Autodesk Fusion 360 part; units mm, degrees
sketch "Sketch1" plane through (0, 0, 0) normal (0, 0, 1) x (1, 0, 0)
  line L0 (0, 0) -> (-200, 0)
  line L1 (-200, 0) -> (-200, 25)
  line L2 (-200, 25) -> (0, 25)
  line L3 (0, 25) -> (0, 0)
extrude "Extrude1" add sketch "Sketch1" along normal blind 30
ref_plane "WorkPlane2" through (-100, 12.5, 15) normal (1, 0, 0) x (0, 1, 0)
sketch "Sketch2" plane through (0, 0, 0) normal (0, -1, 0) x (1, 0, 0)
  line L0 (-200, 0) -> (0, 0)
  line L1 (0, 0) -> (0, 30)
  line L2 (0, 30) -> (-200, 30)
  line L3 (-200, 30) -> (-200, 0)
ref_plane "WorkPlane1" through (-100, 12.5, 15) normal (0, 0, 1) x (1, 0, 0)
sketch "Sketch3" plane through (0, 0, 15) normal (0, 0, 1) x (1, 0, 0)
  line L0 (-200, 25) -> (-180, 25)
  line L1 (-180, 25) -> (-180, 0)
  line L2 (-180, 0) -> (-200, 0)
  line L3 (-200, 0) -> (-200, 25)
extrude "Extrude2" cut 1 faces at (-200, 8.3333, 20) along direction (1, 0, 0) blind 1
sketch "Sketch4" plane through (0, 0, 30) normal (0, 0, 1) x (-1, 0, 0)
  line L0 (0, -25) -> (199, -25)
  line L1 (199, 0) -> (0, 0)
  line L2 (0, 0) -> (22, 0)
  line L3 (22, 0) -> (22, -25)
  line L4 (22, -25) -> (0, -25)
  line L5 (0, -25) -> (0, 0)
  line L6 (199, -25) -> (199, 0)
  line L7 (0, 0) -> (0, -25)
extrude "Extrude3" cut sketch "Sketch4" against normal blind 6 contours L0 L1 L2 L3 L4 L5 L7
sketch "Sketch5" plane through (0, 0, 0) normal (0, 0, -1) x (1, 0, 0)
  line L0 (0, 0) -> (-199, 0)
  line L1 (-199, -25) -> (0, -25)
  line L2 (0, 0) -> (-22, 0)
  line L3 (-22, 0) -> (-22, -25)
  line L4 (-22, -25) -> (0, -25)
  line L5 (0, -25) -> (0, 0)
  line L6 (-199, 0) -> (-199, -25)
  line L7 (0, -25) -> (0, 0)
extrude "Extrude4" cut sketch "Sketch5" against normal blind 6 contours L0 L1 L2 L3 L4 L5 L7
sketch "Sketch6" plane through (0, 0, 30) normal (0, 0, 1) x (-1, 0, 0)
  line L0 (199, 0) -> (22, 0)
  line L1 (22, 0) -> (22, -25)
  line L2 (22, -25) -> (199, -25)
  line L3 (34.9313, -5) -> (165.0687, -5)
  line L4 (165.0687, -5) -> (165.0687, -20)
  line L5 (165.0687, -20) -> (34.9313, -20)
  line L6 (34.9313, -20) -> (34.9313, -5)
  line L7 (199, -25) -> (199, 0)
extrude "Extrude5" cut sketch "Sketch6" against normal blind 43 contours L3 L4 L5 L6
sketch "Sketch7" plane through (0, 25, 0) normal (0, 1, 0) x (-1, 0, 0)
  line L0 (199, 30) -> (22, 30)
  line L1 (22, 30) -> (22, 24)
  line L2 (22, 24) -> (0, 24)
  line L3 (0, 6) -> (22, 6)
  line L4 (22, 6) -> (22, 0)
  line L5 (22, 0) -> (199, 0)
  line L6 (34.8715, 24.9016) -> (165.0188, 24.9016)
  line L7 (165.0188, 24.9016) -> (165.0188, 4.9016)
  line L8 (165.0188, 4.9016) -> (34.8715, 4.9016)
  line L9 (34.8715, 4.9016) -> (34.8715, 24.9016)
  line L10 (199, 0) -> (199, 30)
  line L11 (0, 24) -> (0, 6)
  dimension "d20" = 20
extrude "Extrude6" cut sketch "Sketch7" against normal blind 50 contours L6 L7 L8 L9
sketch "Sketch8" plane through (0, 25, 0) normal (0, 1, 0) x (-1, 0, 0)
sketch "Sketch9" plane through (0, 0, 30) normal (0, 0, 1) x (-1, 0, 0)
  line L0 (165.0687, -5) -> (165.0687, -20)
  line L1 (165.0687, -20) -> (34.9313, -20)
  line L2 (34.9313, -20) -> (34.9313, -5)
  line L3 (34.9313, -5) -> (165.0687, -5)
  line L4 (199, 0) -> (22, 0)
  line L5 (22, 0) -> (22, -25)
  line L6 (22, -25) -> (199, -25)
  line L7 (22, -17.5) -> (37.5, -25)
  line L8 (22, -25) -> (37.5, -25)
  line L9 (22, -25) -> (22, -17.5)
  line L10 (199, -25) -> (199, 0)
ref_plane "WorkPlane3" through (-99.5, 12.5, 15) normal (0, 1, 0) x (-1, 0, 0)
sketch "Sketch10" plane through (0, 0, 30) normal (0, 0, 1) x (-1, 0, 0)
extrude "Extrude7" add 1 faces at (-78.2739, 1.6667, 24.9016) along direction (0, 0, -1) blind 5
extrude "Extrude8" add 1 faces at (-78.2739, 1.6667, 4.9016) along direction (0, 0, 1) blind 5
sketch "Sketch11" plane through (-22, 0, 0) normal (1, 0, 0) x (0, 1, 0)
  line L0 (25, 30) -> (0, 30)
  line L1 (0, 30) -> (0, 24)
  line L2 (0, 24) -> (25, 24)
  line L3 (25, 24) -> (25, 30)
  line L4 (0, 30) -> (25, 30)
  line L5 (25, 30) -> (25, 24)
  line L6 (25, 24) -> (0, 24)
  line L7 (0, 24) -> (0, 30)
  line L8 (0, 6) -> (25, 6)
  line L9 (25, 6) -> (25, 0)
  line L10 (25, 0) -> (0, 0)
  line L11 (0, 0) -> (0, 6)
extrude "Extrude9" cut sketch "Sketch11" against normal blind 220
sketch "Sketch12" plane through (0, 0, 24) normal (0, 0, 1) x (-1, 0, 0)
  line L0 (34.9313, -5) -> (165.0687, -5)
  line L1 (165.0687, -5) -> (165.0687, -20)
  line L2 (165.0687, -20) -> (34.9313, -20)
  line L3 (34.9313, -20) -> (34.9313, -5)
  line L4 (0, -25) -> (199, -25)
  line L5 (199, 0) -> (0, 0)
  line L6 (25, -25) -> (25, 0)
  line L7 (199, -25) -> (199, 0)
  line L8 (0, 0) -> (0, -25)
extrude "Extrude10" add 1 faces at (-187.6729, 0, 16.6339) along direction (0, -1, 0) blind 30
sketch "Sketch13" plane through (0, 0, 24) normal (0, 0, 1) x (-1, 0, 0)
  line L0 (34.9313, -5) -> (165.0687, -5)
  line L1 (165.0687, -5) -> (165.0687, -20)
  line L2 (165.0687, -20) -> (34.9313, -20)
  line L3 (34.9313, -20) -> (34.9313, -5)
  line L4 (0, -25) -> (199, -25)
  line L5 (199, 30) -> (0, 30)
  line L6 (165, -5) -> (35, -5)
  line L7 (35, -5) -> (35, 25)
  line L8 (35, 25) -> (165, 25)
  line L9 (165, 25) -> (165, -5)
  line L10 (35, -5) -> (165, -5)
  line L11 (165, -5) -> (165, 25)
  line L12 (165, 25) -> (35, 25)
  line L13 (35, 25) -> (35, -5)
  line L14 (199, -25) -> (199, 30)
  line L15 (0, 30) -> (0, -25)
sketch "Sketch14" plane through (0, 0, 24) normal (0, 0, 1) x (-1, 0, 0)
  line L0 (34.9313, -5) -> (165.0687, -5)
  line L1 (165.0687, -5) -> (165.0687, -20)
  line L2 (165.0687, -20) -> (34.9313, -20)
  line L3 (34.9313, -20) -> (34.9313, -5)
  line L4 (0, -25) -> (199, -25)
  line L5 (199, 30) -> (0, 30)
  line L6 (165, -5) -> (35, -5)
  line L7 (35, -5) -> (35, 25)
  line L8 (35, 25) -> (165, 25)
  line L9 (165, 25) -> (165, -5)
  line L10 (35, 25) -> (165, 25)
  line L11 (165, 25) -> (165, -5)
  line L12 (165, -5) -> (35, -5)
  line L13 (35, -5) -> (35, 25)
  line L14 (199, -25) -> (199, 30)
  line L15 (0, 30) -> (0, -25)
extrude "Extrude11" cut 1 faces at (-121.6729, 5, 22.6339) along direction (0, -1, 0) blind 30
fillet "Fillet3" radius 25 2 edges at (0, 25, 15) (0, -30, 15)
fillet "Fillet4" radius 25 2 edges at (-199, 25, 15) (-199, -30, 15)
hole "Hole2" at (-13.2303, -1.87, 24) direction (0, 0, -1) diameter 10 depth 40 tip angle 118
scale "Scale1" factor 0.7 about (-34.9313, 20, 24) bodies 1
The model under review builds one solid part; all positions refer to its coordinate system, in mm. A direction names the side the tool comes from. Round coordinates to 2 decimals unless told otherwise and drop trailing zeros. Loops run counter-clockwise (first coordinate to the right, second up) from the corner with the lowest first, then second, coordinate; pieces in that order, holes last. Notation, with made-up numbers: (-18, 81.5) - (12, 81.5) arc R20 cw to (12, 104.5) - close; hole circle Ø6 at (17.5, 19). An arc over 180 degrees is marked (long way). Write each question's results on one line, items separated by ' | '. Start each with the question number.
Q1. Tool access review of faces 5 (the flat face through (-84, 21, 21.131)), 6 (the flat face through (-34.931, 4, 23)), 7 (the cylindrical face through (-15.47, 18.24, 17.79)): name each direction out of +Z, -Z, +X, -X, +Y, -Y from which nothing blocks a thin tool from reaching the whole face with its end or side.
Q2. Take a section at A-A on x = -90. Give the boundary of the cut face in (y, z).
Q3. Draft analysis for pull direction Z (two halves, no side actions). For faces 1 (the flat face through (-81, -13, 24)), 2 (the flat face through (-125.993, 22, 18)), 3 (the flat face through (-149.779, 4, 18)), 4 (the flat face through (-125.993, -13, 18)), state which applies: pulls with the +Z half, pulls with the -Z half, needs draft (parallel to the pull), parting line crosses it, or undercut.
Q4. Take a section at D-D on y = 13. Give the boundary of the cut face in (x, z), plus the area to 3 significant figures.
Q5. Insertion check: P1, Ø1.8, axis at y = -12.5, z = 17, coming from the +X side; P2, Ø6.5, axis at x = -94, z = 15, coming from the +Y side; P3, Ø3, axis at y = 21.5, z = 18.5, coming from the +X side; P4, Ø1, axis at y = -9.5, z = 12.5, coming from the +X side. Each pin has a flat end and moves straight along its axis. Give the tip position at first contact, or say it passes through.
Q6. Wall thickness on line 1 along X through (y, z) = (4.5, 17.75); line 2 along Y through (x, z) = (-42, 12.25); line 3 along Z through (x, y) = (-51, -12): over which ranges is each line inside the solid? List them lowest first. Write a range as [from, to].
Q7. Take a section at C-C on y = -9. Give the boundary of the cut face in (x, z), plus the area to 3 significant figures.
Q8. Take a section at B-B on z = 18. Give the number of separate pieces and of enclosed holes in the cut face, plus the area to 3 significant figures.
Data:
1) face 5: +Y, -Y | face 6: +Z, -Z | face 7: +Z, -Z, +X, +Y
2) outline: (-15, 11.4) - (-11.5, 11.4) - (-11.5, 14.13) - (-15, 14.13) - close; (-15, 21.13) - (-11.5, 21.13) - (-11.5, 24) - (-15, 24) - close; (20, 11.4) - (23.5, 11.4) - (23.5, 14.13) - (20, 14.13) - close; (20, 21.13) - (23.5, 21.13) - (23.5, 24) - (20, 24) - close
3) face 1: pulls with the +Z half | face 2: undercut | face 3: needs draft | face 4: undercut
4) outline: (-148.32, 11.4) - (-126.03, 11.4) - (-126.03, 24) - (-148.32, 24) - close; (-34.93, 11.4) - (-11.94, 11.4) - (-11.94, 24) - (-34.93, 24) - (-34.93, 21.13) - (-34.89, 21.13) - (-34.89, 14.13) - (-34.93, 14.13) - close | area: 570 mm²
5) P1: stops at x = -17.61 | P2: stops at y = 23.5 | P3: stops at x = -17.48 | P4: stops at x = -14.79
6) line 1: x = [-149.78, -126.03], [-34.89, -23.24], [-16.25, -10.48] | line 2: y = [-15, -11.5], [20, 23.5] | line 3: z = [11.4, 14.13], [21.13, 24]
7) outline: (-145.47, 11.4) - (-126.03, 11.4) - (-126.03, 24) - (-145.47, 24) - close; (-34.93, 11.4) - (-14.79, 11.4) - (-14.79, 24) - (-34.93, 24) - (-34.93, 21.13) - (-34.89, 21.13) - (-34.89, 14.13) - (-34.93, 14.13) - close | area: 498 mm²
8) separate pieces: 2 | enclosed holes: 1 | area: 1,550 mm²
